Source: CAD feature listing. Evaluate the final solid. Frame: model axes, mm. A direction names the side the tool comes from. Coordinates: 2 decimals unless noted, no trailing zeros. Loops run counter-clockwise (first coordinate to the right, second up) from the corner with the lowest first, then second, coordinate; pieces in that order, holes last.
Item 1: Section query D-D, the plane x = -23. Return the cut outline in (y, z), then the cut area to 3 significant figures.
Item 2: Reachability of faces 5 (the flat face through (-13.002, 0, -3)), 6 (the flat face through (-39.002, 0, -1)), 7 (the flat face through (-27, 12.899, -3)), 8 (the flat face through (-28, 0, 1.5)), 9 (the flat face through (-27, -12.899, -3)) from +Z, -Z, +X, -X, +Y, -Y: full face, straight path, thin tool, end or side. Return the list, or none.
Item 3: Section query A-A, the plane x = -12. Return the cut outline in (y, z), then the cut area to 3 significant figures.
Item 4: Line query: probe 1 along Y at (x, z) = (34.5, 25.5); probe 2 along Z at (x, y) = (7.5, -5.25); probe 3 along Z at (x, y) = (-27.5, 2.5). Output: solid intervals per line, ascending.
Item 5: Section query B-B, the plane z = 28. Return the cut outline in (x, y).
Item 6: Pin query (flat end, axial travel): pin 1 Ø14 at (x, y) = (11.5, -1.5) entering from -Z; pin 2 Ø14.5 at (y, z) = (-1.5, 22.5) entering from -X; pin 3 Ø8.5 at (y, z) = (6, 15.5) entering from -X. Return the tip coordinate at first contact, or that it passes through.
Item 7: Pull-direction query (Y, two-part tool) for faces 1 (the flat face through (12, -14.158, 16)), 2 (the flat face through (9, 15, 15)), 3 (the flat face through (-1, 0, 0)), 4 (the flat face through (12, 0, 1.497)); classes: +Y half, -Y half, draft (parallel to the pull), parting line (faces both ways), or undercut.
```python
from build123d import *

# Parameters (mm, degrees)
SKETCH_1_W          = 82
SKETCH_1_H          = 30
EXTRUDE_1_DEPTH     = 1.5
SKETCH_2_W          = 1.997612732
SKETCH_2_H          = 25.79850023
EXTRUDE_3_DEPTH     = 3.5
SKETCH_4_W          = 1.75
SKETCH_4_H          = 25.79850023
EXTRUDE_4_DEPTH     = 26
SKETCH_5_W          = 55.064096776
SKETCH_5_H          = 30
EXTRUDE_5_DEPTH     = 29
SKETCH_6_W          = 26.352675357
SKETCH_6_H          = 28.194959652
CUT_EXTRUDE_1_DEPTH = 53
SKETCH_8_W          = 53
SKETCH_8_H          = 28.194959652
CUT_EXTRUDE_2_DEPTH = 1.32


with BuildPart() as part:
    # 草圖1 → 填料-伸長1 (new body)
    with BuildSketch(Plane.XY):
        Rectangle(SKETCH_1_W, SKETCH_1_H)
    extrude(amount=EXTRUDE_1_DEPTH)

    # 草圖2 → 填料-伸長3 (add)
    with BuildSketch(Plane(origin=(0, 0, 0), x_dir=(-1, 0, 0), z_dir=(0, 0, -1))):
        with Locations((40.001193634, 0)):
            Rectangle(SKETCH_2_W, SKETCH_2_H)
    extrude(amount=EXTRUDE_3_DEPTH)

    # 草圖4 → 填料-伸長4 (add)
    with BuildSketch(Plane(origin=(-39.002387268, 0, 0), x_dir=(0, 0, -1), z_dir=(1, 0, 0))):
        with Locations((2.625, 0)):
            Rectangle(SKETCH_4_W, SKETCH_4_H)
    extrude(amount=EXTRUDE_4_DEPTH)

    # 草圖5 → 填料-伸長5 (add)
    with BuildSketch(Plane.XY.offset(1.5)):
        with Locations((13.467951612, 0)):
            Rectangle(SKETCH_5_W, SKETCH_5_H)
    extrude(amount=EXTRUDE_5_DEPTH)

    # 草圖6 → 除料-伸長1 (cut)
    with BuildSketch(Plane.ZY.offset(14.064096776)):
        with Locations((15.993727328, -0.060074488)):
            Rectangle(SKETCH_6_W, SKETCH_6_H)
    extrude(amount=-CUT_EXTRUDE_1_DEPTH, mode=Mode.SUBTRACT)

    # 草圖8 → 除料-伸長2 (cut)
    with BuildSketch(Plane.XY.offset(2.817389649)):
        with Locations((12.435903224, -0.060074488)):
            Rectangle(SKETCH_8_W, SKETCH_8_H)
    extrude(amount=-CUT_EXTRUDE_2_DEPTH, mode=Mode.SUBTRACT)


solid = part.part
```
Verdict:
1. outline: (-15, 0) - (15, 0) - (15, 1.5) - (-15, 1.5) - close; (-12.9, -3.5) - (12.9, -3.5) - (12.9, -1.75) - (-12.9, -1.75) - close
1. area: 90.1 mm2
2. face 5: -Z, +X, +Y, -Y
2. face 6: +X, +Y, -Y
2. face 7: -Z, +X, -X, +Y
2. face 8: +Z, -X, +Y, -Y
2. face 9: -Z, +X, -X, -Y
3. outline: (-15, 0) - (15, 0) - (15, 30.5) - (-15, 30.5) - close; hole (-14.16, 1.5) - (14.04, 1.5) - (14.04, 29.17) - (-14.16, 29.17) - close
3. area: 135 mm2
4. probe 1: y = -15 to -14.16, 14.04 to 15
4. probe 2: z = 0 to 1.5, 29.17 to 30.5
4. probe 3: z = -3.5 to -1.75, 0 to 1.5
5. outline: (-14.06, -15) - (41, -15) - (41, 15) - (-14.06, 15) - (-14.06, 14.04) - (38.94, 14.04) - (38.94, -14.16) - (-14.06, -14.16) - close
6. pin 1: stops at z = 0
6. pin 2: stops at x = -14.06
6. pin 3: stops at x = 38.94
7. face 1: undercut
7. face 2: +Y half
7. face 3: draft
7. face 4: undercut
